The listing builds one solid part. Answer for the finished solid, in the listing's coordinates (mm). Face numbers are marked on the shaded views. Coordinates: 2 decimals unless noted, no trailing zeros. Order: outer loops, then holes, each group sorted by start corner. A loop starts at its lowest first (then second) coordinate and runs counter-clockwise, first axis right, second up.
Autodesk Inventor part; units mm, degrees
ref_plane "YZ Plane" through (0, 0, 0) normal (1, 0, 0) x (0, 1, 0)
ref_plane "XZ Plane" through (0, 0, 0) normal (0, 1, 0) x (-1, 0, 0)
ref_plane "XY Plane" through (0, 0, 0) normal (0, 0, 1) x (1, 0, 0)
sketch "Sketch1" plane through (0, 0, 0) normal (0, 0, 1) x (1, 0, 0)
  circle A0 centre (0, 0) radius 3
  line L0 (0, 0) -> (0, 6) construction
  line L1 (0, 6) -> (0, -6) construction
  line L2 (0, -6) -> (5, -6)
  line L3 (7, -4) -> (7, 4)
  line L4 (5, 6) -> (0, 6)
  line L5 (0, 6) -> (-11, 6)
  line L6 (-15, 2) -> (-15, -2)
  line L7 (-11, -6) -> (0, -6)
  arc A1 (7, 4) -> (5, 6) centre (5, 4) ccw
  arc A2 (5, -6) -> (7, -4) centre (5, -4) ccw
  arc A3 (-11, 6) -> (-15, 2) centre (-11, 2) ccw
  arc A4 (-15, -2) -> (-11, -6) centre (-11, -2) ccw
  line L8 (0, 0) -> (9, 0) construction
  line L9 (9, 0) -> (9, 8.7977) construction
  point P0 (7, -6)
  point P1 (-15, 6)
  dimension "d0" = 6
  dimension "d1" = 6
  dimension "d2" = 12
  dimension "d3" = 7
  dimension "d4" = 15
  dimension "d5" = 2
  dimension "d6" = 4
  dimension "d7" = 4
  dimension "d16" = 9
extrude "Extrusion1" add sketch "Sketch1" along normal blind 8
sketch "Sketch3" plane through (-15, -2, 0) normal (-1, 0, 0) x (0, 0, 1)
  line L0 (0, 2) -> (4, 2) construction
  circle A0 centre (4, 2) radius 2.5
  dimension "d17" = 4
  dimension "d18" = 5
extrude "Extrusion3" cut sketch "Sketch3" against normal blind 8
thread "Thread2"
equation "\"BendRadius\" = Thickness"
equation "\"BendReliefWidth\" = Thickness"
equation "\"BendReliefDepth\" = 0.5 * Thickness"
equation "\"CornerReliefSize\" = 4 * Thickness"
equation "\"MinimumRemnant\" = 2 * Thickness"
equation "\"TransitionRadius\" = BendRadius"
equation "\"JacobiRadiusSize\" = BendRadius"
equation "\"GapSize\" = Thickness"
properties part number "Mocowanie przesuwnicy" material "Stainless Steel"
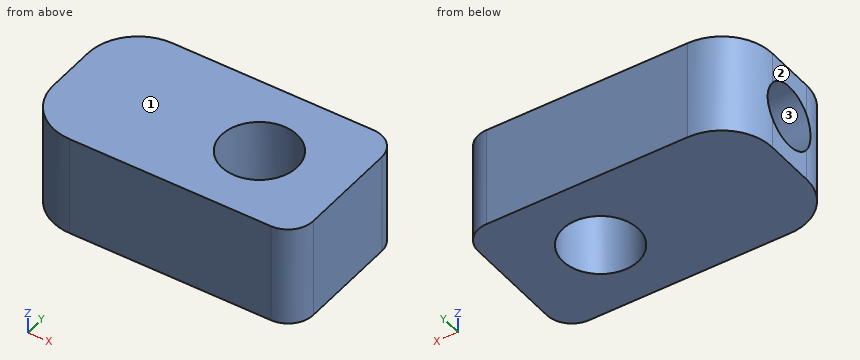
1) A cutting plane is placed at B-B, the plane y = 0. Write down the section's boundary in (x, z).
2) A cutting plane is placed at C-C, the plane z = 4. Write down the section's boundary in (x, y).
3) The mould has two halves that part along Z. Classify the marked faces 1, 2 and 3: released by +Z, released by -Z, zero draft, split by the parting line, or undercut.
4) A cutting plane is placed at D-D, the plane x = -9.5. Write down the section's boundary in (y, z), plus the area to 3 significant figures.
5) A cutting plane is placed at A-A, the plane x = 0. Write down the section's boundary in (y, z).
6) Straight lines are drawn through the part: probe 1 along Y at (x, z) = (-10.75, 4); probe 2 along Z at (x, y) = (-11.75, -2); probe 3 along Y at (x, z) = (-10.5, 5.25). For each, find the intervals that lie inside material, in ascending order.
Working result:
1. outline: (-15, 0) - (-3, 0) - (-3, 8) - (-15, 8) - (-15, 6.5) - (-7, 6.5) - (-7, 1.5) - (-15, 1.5) - close; (3, 0) - (7, 0) - (7, 8) - (3, 8) - close
2. outline: (-14.97, -2.5) arc R4 ccw to (-11, -6) - (5, -6) arc R2 ccw to (7, -4) - (7, 4) arc R2 ccw to (5, 6) - (-11, 6) arc R4 ccw to (-14.97, 2.5) - (-7, 2.5) - (-7, -2.5) - close; hole circle Ø6 at (0, 0)
3. face 1: released by +Z
3. face 2: zero draft
3. face 3: undercut
4. outline: (-6, 0) - (6, 0) - (6, 8) - (-6, 8) - close; hole circle Ø5 at (0, 4)
4. area: 76.4 mm2
5. outline: (-6, 0) - (-3, 0) - (-3, 8) - (-6, 8) - close; (3, 0) - (6, 0) - (6, 8) - (3, 8) - close
6. probe 1: y = -6 to -2.5, 2.5 to 6
6. probe 2: z = 0 to 2.5, 5.5 to 8
6. probe 3: y = -6 to -2.17, 2.17 to 6
